Part print with two shaded views. Sizes in mm from the minimum x, y, z corner. A direction names the side the tool comes from. Round coordinates to 2 decimals unless told otherwise and drop trailing zeros. Write each loop counter-clockwise with the first axis right and the second up, starting at its lowest first coordinate (ties: lowest second). Pieces come first, ordered by that corner, then holes. Notation, with made-up numbers: (62.25, -34.75) -> (112.25, -34.75) arc R8 ccw to (112.25, -26.75) -> close; hole circle Ø7 at (7.25, 60.25). An arc over 180 degrees is marked (long way). Return JSON: item names as keys, results as strings.
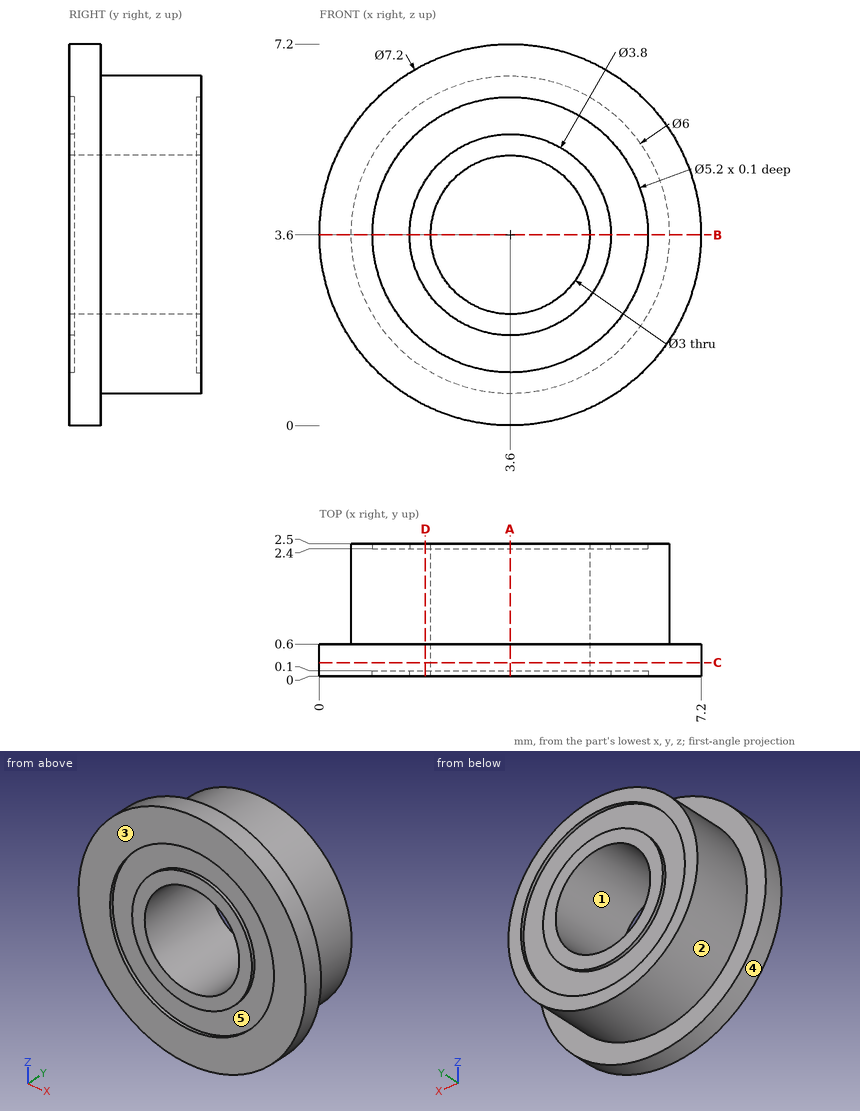
Q1. Wall check: L1, parallel to Z at x = 3.6, y = 2.45; L2, parallel to Z at x = 3.6, y = 0.05; L3, parallel to X at y = 1.3, z = 4. Give the ranges that are in metal, low to high.
Verdict:
{"L1": "z = 0.6 to 1, 1.7 to 2.1, 5.1 to 5.5, 6.2 to 6.6", "L2": "z = 0 to 1, 1.7 to 2.1, 5.1 to 5.5, 6.2 to 7.2", "L3": "x = 0.63 to 2.15, 5.05 to 6.57"}
Q2. 3-axis set-ups, long thin cutter, end or side, ignore diameter. For the marked faces 1 and 2: which of +Z, -Z, +X, -X, +Y, -Y reach the whole face in a straight line?
Verdict:
{"face 1": "+Y, -Y", "face 2": "+Y"}
Q3. Pin check, flat tip, straight feed: pin 1 Ø1.5 at (x, y) = (5, 2) entering from +Z. Stop position of the tip, or through.
Verdict:
{"pin 1": "stops at z = 6.53"}
Q4. Saw through at B-B on z = 3.6. List the corners of the cut face in (x, y).
Verdict:
{"outline": "(0, 0) -> (1, 0) -> (1, 0.1) -> (1.7, 0.1) -> (1.7, 0) -> (2.1, 0) -> (2.1, 2.5) -> (1.7, 2.5) -> (1.7, 2.4) -> (1, 2.4) -> (1, 2.5) -> (0.6, 2.5) -> (0.6, 0.6) -> (0, 0.6) -> close; (5.1, 0) -> (5.5, 0) -> (5.5, 0.1) -> (6.2, 0.1) -> (6.2, 0) -> (7.2, 0) -> (7.2, 0.6) -> (6.6, 0.6) -> (6.6, 2.5) -> (6.2, 2.5) -> (6.2, 2.4) -> (5.5, 2.4) -> (5.5, 2.5) -> (5.1, 2.5) -> close"}
Q5. Two-plate mould, pull along Z, no slides. Class the marked faces 3, 4 and 5: +Z half, -Z half, draft (parallel to the pull), parting line (faces both ways), or undercut.
Verdict:
{"face 3": "draft", "face 4": "parting line", "face 5": "undercut"}
Q6. Saw through at A-A on x = 3.6. List the corners of the cut face in (y, z), then the cut area to 3 significant figures.
Verdict:
{"outline": "(0, 0) -> (0.6, 0) -> (0.6, 0.6) -> (2.5, 0.6) -> (2.5, 1) -> (2.4, 1) -> (2.4, 1.7) -> (2.5, 1.7) -> (2.5, 2.1) -> (0, 2.1) -> (0, 1.7) -> (0.1, 1.7) -> (0.1, 1) -> (0, 1) -> close; (0, 5.1) -> (2.5, 5.1) -> (2.5, 5.5) -> (2.4, 5.5) -> (2.4, 6.2) -> (2.5, 6.2) -> (2.5, 6.6) -> (0.6, 6.6) -> (0.6, 7.2) -> (0, 7.2) -> (0, 6.2) -> (0.1, 6.2) -> (0.1, 5.5) -> (0, 5.5) -> close", "area": "7.94 mm²"}
Q7. Saw through at C-C on y = 0.25. List the corners of the cut face in (x, z), then the cut area to 3 significant figures.
Verdict:
{"outline": "circle Ø7.2 at (3.6, 3.6); hole circle Ø3 at (3.6, 3.6)", "area": "33.6 mm²"}
Q8. Saw through at D-D on x = 2. List the corners of the cut face in (y, z), then the cut area to 3 significant figures.
Verdict:
{"outline": "(0, 0.38) -> (0.6, 0.38) -> (0.6, 1.06) -> (2.5, 1.06) -> (2.5, 1.55) -> (2.4, 1.55) -> (2.4, 2.58) -> (2.5, 2.58) -> (2.5, 4.62) -> (2.4, 4.62) -> (2.4, 5.65) -> (2.5, 5.65) -> (2.5, 6.14) -> (0.6, 6.14) -> (0.6, 6.82) -> (0, 6.82) -> (0, 5.65) -> (0.1, 5.65) -> (0.1, 4.62) -> (0, 4.62) -> (0, 2.58) -> (0.1, 2.58) -> (0.1, 1.55) -> (0, 1.55) -> close", "area": "13.1 mm²"}
